For this review, take the finished solid that the model builds, in its own axes (mm). Coordinates: 2 decimals unless noted, no trailing zeros. Write each loop counter-clockwise with the first axis right and the second up, starting at its lowest first coordinate (ties: lowest second). Pieces come first, ordered by that corner, then holes.
1) To check wall thickness, follow line 1 along Y through (x, z) = (-13.5, 1385). State the ranges of the line that lie inside material, in increasing order.
2) We need section A-A on x = 2. Write out the cut boundary in (y, z), then the cut area to 3 significant figures.
3) Insertion check: P1, Ø5, axis at x = -11.5, y = -6, coming from the +Z side. The pin has a flat end and moves straight along its axis. Give the tip position at first contact, or say it passes through.
4) We need section C-C on z = 569. Write out the cut boundary in (x, y), then the cut area to 3 significant figures.
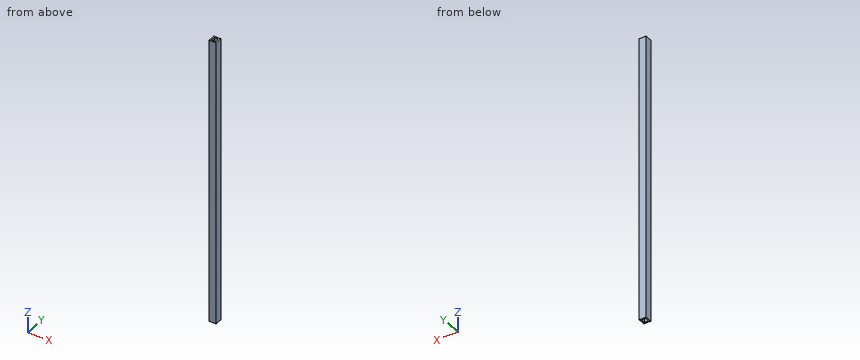
from build123d import *

# Parameters (mm, degrees)
SKETCH1_W                 = 50
SKETCH1_H                 = 50
SKETCH1_W_2               = 30
SKETCH1_H_2               = 30
BOSS_EXTRUDE1_DEPTH       = 2100
SKETCH2_W                 = 50
SKETCH2_H                 = 50
BOSS_EXTRUDE2_DEPTH       = 5100
SKETCH4_W                 = 50
SKETCH4_H                 = 50
SKETCH4_W_2               = 30
SKETCH4_H_2               = 30
BOSS_EXTRUDE3_DEPTH       = 2100
SKETCH5_W                 = 50
SKETCH5_H                 = 50
BOSS_EXTRUDE4_DEPTH       = 1800
LPATTERN1_COUNT           = 2
LPATTERN1_PITCH           = 2000
SKETCH6_W                 = 100
SKETCH6_H                 = 150
BOSS_EXTRUDE5_DEPTH       = 5
SKETCH7_W                 = 100
SKETCH7_H                 = 150
BOSS_EXTRUDE6_DEPTH       = 5
SKETCH8_W                 = 100
SKETCH8_H                 = 150
BOSS_EXTRUDE7_DEPTH       = 5
SKETCH9_W                 = 100
SKETCH9_H                 = 150
BOSS_EXTRUDE8_DEPTH       = 5
SKETCH10_W                = 100
SKETCH10_H                = 5
BOSS_EXTRUDE9_DEPTH       = 20
SKETCH11_W                = 100
SKETCH11_H                = 5
BOSS_EXTRUDE10_DEPTH      = 20
SKETCH12_W                = 100
SKETCH12_H                = 5
BOSS_EXTRUDE11_DEPTH      = 20
SKETCH13_W                = 100
SKETCH13_H                = 5
BOSS_EXTRUDE12_DEPTH      = 20
F_5_0MM_DOWEL_HOLE1_D     = 5
F_5_0MM_DOWEL_HOLE1_DEPTH = 20
F_5_0MM_DOWEL_HOLE1_TIP   = 1.502151548
F_5_0MM_DOWEL_HOLE2_D     = 5
F_5_0MM_DOWEL_HOLE2_DEPTH = 20
F_5_0MM_DOWEL_HOLE2_TIP   = 1.502151548
F_5_0MM_DOWEL_HOLE3_D     = 5
F_5_0MM_DOWEL_HOLE3_DEPTH = 20
F_5_0MM_DOWEL_HOLE3_TIP   = 1.502151548
F_5_0MM_DOWEL_HOLE4_D     = 5
F_5_0MM_DOWEL_HOLE4_DEPTH = 20
F_5_0MM_DOWEL_HOLE4_TIP   = 1.502151548
SKETCH26_W                = 5305.980467783
SKETCH26_H                = 67.779411833
CUT_EXTRUDE1_DEPTH        = 5613.586302232
SPLIT1_OUTLINE_W          = 5150
SPLIT1_OUTLINE_H          = 50
SPLIT1_OUTLINE_W_2        = 30
SPLIT1_OUTLINE_H_2        = 30
SPLIT1_DEPTH              = 2100
SPLIT1_START              = -5
SPLIT1_2_OUTLINE_W        = 100
SPLIT1_2_OUTLINE_H        = 120
SPLIT1_2_OUTLINE_R        = 2.5
SPLIT1_2_DEPTH            = 2110
SPLIT3_START              = -5
SPLIT3_OUTLINE_W          = 100
SPLIT3_OUTLINE_H          = 120
SPLIT3_OUTLINE_R          = 2.5
SPLIT3_DEPTH              = 5
SPLIT4_START              = 2100
SPLIT4_OUTLINE_W          = 100
SPLIT4_OUTLINE_H          = 120
SPLIT4_OUTLINE_R          = 2.5
SPLIT4_DEPTH              = 5


# Read off the part's stored shape, not the designer's step: Split1, Split3, Split4
with BuildPart() as part:
    # Sketch1 → Boss-Extrude1 (new body)
    with BuildSketch(Plane.XY):
        Rectangle(SKETCH1_W, SKETCH1_H)
        Rectangle(SKETCH1_W_2, SKETCH1_H_2, mode=Mode.SUBTRACT)
    extrude(amount=BOSS_EXTRUDE1_DEPTH)

    # Sketch2 → Boss-Extrude2 (add)
    with BuildSketch(Plane.ZY.offset(25)):
        with Locations((125, 0)):
            Rectangle(SKETCH2_W, SKETCH2_H)
        with Locations((1975, 0)):
            Rectangle(SKETCH2_W, SKETCH2_H)
    extrude(amount=BOSS_EXTRUDE2_DEPTH)

    # Sketch4 → Boss-Extrude3 (add)
    with BuildSketch(Plane.XY):
        with Locations((-5150, 0)):
            Rectangle(SKETCH4_W, SKETCH4_H)
        with Locations((-5150, 0)):
            Rectangle(SKETCH4_W_2, SKETCH4_H_2, mode=Mode.SUBTRACT)
    extrude(amount=BOSS_EXTRUDE3_DEPTH)

    # Sketch5 → Boss-Extrude4 (add)
    with BuildSketch(Plane(origin=(0, 0, 1950), x_dir=(-1, 0, 0), z_dir=(0, 0, -1))):
        with Locations((1550, 0)):
            Rectangle(SKETCH5_W, SKETCH5_H)
    boss_extrude4 = extrude(amount=BOSS_EXTRUDE4_DEPTH)

    # LPattern1: Boss-Extrude4 ×2
    with Locations(*[(-i * LPATTERN1_PITCH, 0, 0) for i in range(1, LPATTERN1_COUNT)]):
        add(boss_extrude4)

    # Sketch6 → Boss-Extrude5 (add)
    with BuildSketch(Plane(origin=(0, 0, 0), x_dir=(-1, 0, 0), z_dir=(0, 0, -1))):
        Rectangle(SKETCH6_W, SKETCH6_H)
    extrude(amount=BOSS_EXTRUDE5_DEPTH)

    # Sketch7 → Boss-Extrude6 (add)
    with BuildSketch(Plane(origin=(0, 0, 0), x_dir=(-1, 0, 0), z_dir=(0, 0, -1))):
        with Locations((5150, 0)):
            Rectangle(SKETCH7_W, SKETCH7_H)
    extrude(amount=BOSS_EXTRUDE6_DEPTH)

    # Sketch8 → Boss-Extrude7 (add)
    with BuildSketch(Plane.XY.offset(2100)):
        with Locations((-5150, 0)):
            Rectangle(SKETCH8_W, SKETCH8_H)
    extrude(amount=BOSS_EXTRUDE7_DEPTH)

    # Sketch9 → Boss-Extrude8 (add)
    with BuildSketch(Plane.XY.offset(2100)):
        Rectangle(SKETCH9_W, SKETCH9_H)
    extrude(amount=BOSS_EXTRUDE8_DEPTH)

    # Sketch10 → Boss-Extrude9 (add)
    with BuildSketch(Plane(origin=(0, 75, 0), x_dir=(1, 0, 0), z_dir=(0, 1, 0))):
        with Locations((0, -2102.5)):
            Rectangle(SKETCH10_W, SKETCH10_H)
    extrude(amount=BOSS_EXTRUDE9_DEPTH)

    # Sketch11 → Boss-Extrude10 (add)
    with BuildSketch(Plane(origin=(0, 75, 0), x_dir=(1, 0, 0), z_dir=(0, 1, 0))):
        with Locations((0, 2.5)):
            Rectangle(SKETCH11_W, SKETCH11_H)
    extrude(amount=BOSS_EXTRUDE10_DEPTH)

    # Sketch12 → Boss-Extrude11 (add)
    with BuildSketch(Plane(origin=(0, 75, 0), x_dir=(1, 0, 0), z_dir=(0, 1, 0))):
        with Locations((-5150, 2.5)):
            Rectangle(SKETCH12_W, SKETCH12_H)
    extrude(amount=BOSS_EXTRUDE11_DEPTH)

    # Sketch13 → Boss-Extrude12 (add)
    with BuildSketch(Plane(origin=(0, 75, 0), x_dir=(1, 0, 0), z_dir=(0, 1, 0))):
        with Locations((-5150, -2102.5)):
            Rectangle(SKETCH13_W, SKETCH13_H)
    extrude(amount=BOSS_EXTRUDE12_DEPTH)

    # Ø5.0mm Dowel Hole1
    with Locations(Plane(origin=(0, 0, -5), x_dir=(-1, 0, 0), z_dir=(0, 0, -1))):
        with Locations((5110, 75), (5190, 75), (5190, -15), (5110, -15)):
            Hole(F_5_0MM_DOWEL_HOLE1_D / 2, depth=F_5_0MM_DOWEL_HOLE1_DEPTH)
            with Locations((0, 0, -(F_5_0MM_DOWEL_HOLE1_DEPTH + F_5_0MM_DOWEL_HOLE1_TIP / 2))):  # 118° drill point
                Cone(0, F_5_0MM_DOWEL_HOLE1_D / 2, F_5_0MM_DOWEL_HOLE1_TIP, mode=Mode.SUBTRACT)

    # Ø5.0mm Dowel Hole2
    with Locations(Plane(origin=(0, 0, -5), x_dir=(-1, 0, 0), z_dir=(0, 0, -1))):
        with Locations((-40, -15), (-40, 75), (40, 75), (40, -15)):
            Hole(F_5_0MM_DOWEL_HOLE2_D / 2, depth=F_5_0MM_DOWEL_HOLE2_DEPTH)
            with Locations((0, 0, -(F_5_0MM_DOWEL_HOLE2_DEPTH + F_5_0MM_DOWEL_HOLE2_TIP / 2))):  # 118° drill point
                Cone(0, F_5_0MM_DOWEL_HOLE2_D / 2, F_5_0MM_DOWEL_HOLE2_TIP, mode=Mode.SUBTRACT)

    # Ø5.0mm Dowel Hole3
    with Locations(Plane.XY.offset(2105)):
        with Locations((-40, -15), (-40, 75), (40, 75), (40, -15)):
            Hole(F_5_0MM_DOWEL_HOLE3_D / 2, depth=F_5_0MM_DOWEL_HOLE3_DEPTH)
            with Locations((0, 0, -(F_5_0MM_DOWEL_HOLE3_DEPTH + F_5_0MM_DOWEL_HOLE3_TIP / 2))):  # 118° drill point
                Cone(0, F_5_0MM_DOWEL_HOLE3_D / 2, F_5_0MM_DOWEL_HOLE3_TIP, mode=Mode.SUBTRACT)

    # Ø5.0mm Dowel Hole4
    with Locations(Plane.XY.offset(2105)):
        with Locations((-5190, 75), (-5110, 75), (-5110, -15), (-5190, -15)):
            Hole(F_5_0MM_DOWEL_HOLE4_D / 2, depth=F_5_0MM_DOWEL_HOLE4_DEPTH)
            with Locations((0, 0, -(F_5_0MM_DOWEL_HOLE4_DEPTH + F_5_0MM_DOWEL_HOLE4_TIP / 2))):  # 118° drill point
                Cone(0, F_5_0MM_DOWEL_HOLE4_D / 2, F_5_0MM_DOWEL_HOLE4_TIP, mode=Mode.SUBTRACT)

    # Sketch26 → Cut-Extrude1 (cut, through all)
    with BuildSketch(Plane.XY.offset(2105)):
        with Locations((-2547.009766109, -58.889705917)):
            Rectangle(SKETCH26_W, SKETCH26_H)
    extrude(amount=-CUT_EXTRUDE1_DEPTH, mode=Mode.SUBTRACT)

    # Split1 outline → Split1 (cut)
    with BuildSketch(Plane.XY):
        with Locations((-2600, 0)):
            Rectangle(SPLIT1_OUTLINE_W, SPLIT1_OUTLINE_H)
        with Locations((-5150, 0)):
            Rectangle(SPLIT1_OUTLINE_W_2, SPLIT1_OUTLINE_H_2, mode=Mode.SUBTRACT)
    extrude(amount=SPLIT1_DEPTH, mode=Mode.SUBTRACT)

    # Split1 2 outline → Split1 2 (cut)
    with BuildSketch(Plane.XY.offset(SPLIT1_START)):
        with Locations((-5150, 35)):
            Rectangle(SPLIT1_2_OUTLINE_W, SPLIT1_2_OUTLINE_H)
        with Locations((-5190, -15)):
            Circle(SPLIT1_2_OUTLINE_R, mode=Mode.SUBTRACT)
        with Locations((-5190, 75)):
            Circle(SPLIT1_2_OUTLINE_R, mode=Mode.SUBTRACT)
        with Locations((-5110, 75)):
            Circle(SPLIT1_2_OUTLINE_R, mode=Mode.SUBTRACT)
        with Locations((-5110, -15)):
            Circle(SPLIT1_2_OUTLINE_R, mode=Mode.SUBTRACT)
    extrude(amount=SPLIT1_2_DEPTH, mode=Mode.SUBTRACT)

    # Split3 outline → Split3 (cut)
    with BuildSketch(Plane.XY.offset(SPLIT3_START)):
        with Locations((0, 35)):
            Rectangle(SPLIT3_OUTLINE_W, SPLIT3_OUTLINE_H)
        with Locations((-40, -15)):
            Circle(SPLIT3_OUTLINE_R, mode=Mode.SUBTRACT)
        with Locations((40, -15)):
            Circle(SPLIT3_OUTLINE_R, mode=Mode.SUBTRACT)
        with Locations((-40, 75)):
            Circle(SPLIT3_OUTLINE_R, mode=Mode.SUBTRACT)
        with Locations((40, 75)):
            Circle(SPLIT3_OUTLINE_R, mode=Mode.SUBTRACT)
    extrude(amount=SPLIT3_DEPTH, mode=Mode.SUBTRACT)

    # Split4 outline → Split4 (cut)
    with BuildSketch(Plane.XY.offset(SPLIT4_START)):
        with Locations((0, 35)):
            Rectangle(SPLIT4_OUTLINE_W, SPLIT4_OUTLINE_H)
        with Locations((-40, -15)):
            Circle(SPLIT4_OUTLINE_R, mode=Mode.SUBTRACT)
        with Locations((40, -15)):
            Circle(SPLIT4_OUTLINE_R, mode=Mode.SUBTRACT)
        with Locations((-40, 75)):
            Circle(SPLIT4_OUTLINE_R, mode=Mode.SUBTRACT)
        with Locations((40, 75)):
            Circle(SPLIT4_OUTLINE_R, mode=Mode.SUBTRACT)
    extrude(amount=SPLIT4_DEPTH, mode=Mode.SUBTRACT)


solid = part.part
Result:
1. line 1: y = -25 to -15, 15 to 25
2. outline: (-25, 0) - (-15, 0) - (-15, 2100) - (-25, 2100) - close; (15, 0) - (25, 0) - (25, 2100) - (15, 2100) - close
2. area: 42,000 mm2
3. P1: passes through
4. outline: (-25, -25) - (25, -25) - (25, 25) - (-25, 25) - close; hole (-15, -15) - (15, -15) - (15, 15) - (-15, 15) - close
4. area: 1,600 mm2
